from build123d import *

# Parameters (mm, degrees)
F0_R     = 36.5
F0_R_2   = 32.05
F1_DEPTH = 15.875
F2_SIZE  = 0.762
F3_SIZE  = 2.54


with BuildPart() as f1:
    # F0 (on Right) → F1 (new body)
    with BuildSketch(Plane.YZ):
        Circle(F0_R)
        Circle(F0_R_2, mode=Mode.SUBTRACT)
    extrude(amount=F1_DEPTH)

    # F2
    f2_edges = [f1.edges().sort_by_distance(p)[0] for p in [
        (15.875, -36.5, 0),
    ]]
    chamfer(f2_edges, length=F2_SIZE)

    # F3
    f3_edges = [f1.edges().sort_by_distance(p)[0] for p in [
        (0, -32.05, 0),
    ]]
    chamfer(f3_edges, length=F3_SIZE)


solid = f1.part
For this review, take the finished solid that the model builds, in its own axes (mm). Give positions to 0.01 mm unless a question says otherwise; leave off trailing zeros. Loops run counter-clockwise (first coordinate to the right, second up) from the corner with the lowest first, then second, coordinate; pieces in that order, holes last. Notation, with made-up numbers: M -13,81.25 L 12,81.25 A14 cw 12,97.25 Z; hole C -17.5,75 d6. An arc over 180 degrees is marked long. Put each result on its own line as item: value. Start each with the question number.
(1) Add section C-C, the plane x = 9.25. Write out the cut boundary in (y, z), then the cut area to 3 significant figures.
(2) Wall thickness on L1, parallel to Z at x = 7, y = 0; L2, parallel to Y at x = 7.25, z = 1; L3, parallel to Y at x = 4.25, z = -7.5: over which ranges is each line inside the solid? List them lowest first.
(3) For pin 1 (6 mm diameter, centred on x = 3.5, y = -7, fed in from -Z); pin 2 (5 mm diameter, centred on x = 2, z = 22, fed in from +Y); pin 3 (3 mm diameter, centred on y = -17, z = -27.5, fed in from -X), all flat-tipped, find the tip position at first contact; note any pin that passes through.
(4) Add section A-A, the plane z = 0. Write out the cut boundary in (x, y) (3 decimals), then the cut area to 3 significant figures.
(5) The part is to be moulded in two halves that separate along Z. For faces 1 (the conical face through (2.417, -4.188, 31.9)), 2 (the cylindrical face through (7.451, -7.912, -35.632)), 3 (the flat face through (0, -22, -27)), say which applies: +Z half, -Z half, draft (parallel to the pull), parting line (faces both ways), or undercut.
Result:
1. outline: C 0,0 d73; hole C 0,0 d64.1
1. area: 958 mm^2
2. L1: z = -36.5 to -32.05, 32.05 to 36.5
2. L2: y = -36.49 to -32.03, 32.03 to 36.49
2. L3: y = -35.72 to -31.16, 31.16 to 35.72
3. pin 1: stops at z = -36.28
3. pin 2: stops at y = 30.85
3. pin 3: stops at x = 0.76
4. outline: M 0,-36.5 L 15.113,-36.5 L 15.875,-35.738 L 15.875,-32.05 L 2.54,-32.05 L 0,-34.59 Z; M 0,34.59 L 2.54,32.05 L 15.875,32.05 L 15.875,35.738 L 15.113,36.5 L 0,36.5 Z
4. area: 134 mm^2
5. face 1: undercut
5. face 2: parting line
5. face 3: draft
